```python
from build123d import *

# Parameters (mm, degrees)
SKETCH1_W           = 200
SKETCH1_H           = 42
BOSS_EXTRUDE1_DEPTH = 6.35
SKETCH4_R           = 2.286
CUT_EXTRUDE3_DEPTH  = 7.35
CHAMFER1_SIZE       = 5
SKETCH9_R           = 11
CUT_EXTRUDE8_DEPTH  = 7.35
SKETCH12_R          = 2.286
CUT_EXTRUDE11_DEPTH = 7.35
SKETCH13_R          = 2.286
SKETCH13_R_2        = 2.54
CUT_EXTRUDE12_DEPTH = 10


with BuildPart() as part:
    # Sketch1 → Boss-Extrude1 (new body)
    with BuildSketch(Plane.XY):
        Rectangle(SKETCH1_W, SKETCH1_H)
    extrude(amount=BOSS_EXTRUDE1_DEPTH)

    # Sketch4 → Cut-Extrude3 (cut, through all)
    with BuildSketch(Plane.XY.offset(6.35)):
        with Locations((-76, 0)):
            Circle(SKETCH4_R)
    extrude(amount=-CUT_EXTRUDE3_DEPTH, mode=Mode.SUBTRACT)

    # Chamfer1
    chamfer1_edges = [part.edges().sort_by_distance(p)[0] for p in [
        (100, -21, 3.175),
        (-100, -21, 3.175),
        (-100, 21, 3.175),
        (100, 21, 3.175),
    ]]
    chamfer(chamfer1_edges, length=CHAMFER1_SIZE)

    # Sketch9 → Cut-Extrude8 (cut, through all)
    with BuildSketch(Plane.XY.offset(6.35)):
        with Locations((80, 0)):
            Circle(SKETCH9_R)
    extrude(amount=-CUT_EXTRUDE8_DEPTH, mode=Mode.SUBTRACT)

    # Sketch12 → Cut-Extrude11 (cut, through all)
    with BuildSketch(Plane.XY.offset(6.35)):
        with Locations((-93, 0)):
            Circle(SKETCH12_R)
    extrude(amount=-CUT_EXTRUDE11_DEPTH, mode=Mode.SUBTRACT)

    # Sketch13 → Cut-Extrude12 (cut)
    with BuildSketch(Plane.XY.offset(6.35)):
        Polygon((-50, -16), (-50, 16), (-45, 21), (-95, 21), (-100, 16), (-100, -16), (-95, -21), (-45, -21), align=None)
        with Locations((-93, 0)):
            Circle(SKETCH13_R, mode=Mode.SUBTRACT)
        with Locations((-76, 0)):
            Circle(SKETCH13_R, mode=Mode.SUBTRACT)
        with Locations((-35, 10)):
            Circle(SKETCH13_R_2)
        with Locations((-35, -10)):
            Circle(SKETCH13_R_2)
        with Locations((-20, 10)):
            Circle(SKETCH13_R_2)
        with Locations((-20, -10)):
            Circle(SKETCH13_R_2)
        with Locations((-5, 10)):
            Circle(SKETCH13_R_2)
        with Locations((-5, -10)):
            Circle(SKETCH13_R_2)
        with Locations((10, 10)):
            Circle(SKETCH13_R_2)
        with Locations((10, -10)):
            Circle(SKETCH13_R_2)
    extrude(amount=-CUT_EXTRUDE12_DEPTH, mode=Mode.SUBTRACT)


solid = part.part
```
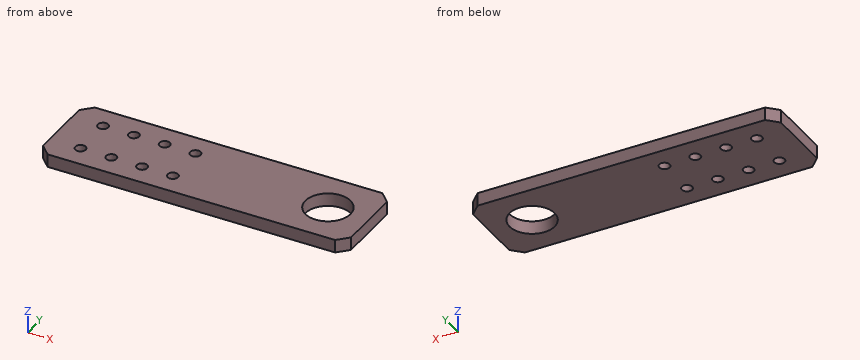
Work out the finished part from the listing and answer in its coordinate system (mm). Give positions to 0.01 mm unless a question says otherwise; leave off trailing zeros. Loops run counter-clockwise (first coordinate to the right, second up) from the corner with the lowest first, then second, coordinate; pieces in that order, holes last. Notation, with made-up numbers: (31.25, 9.5) -> (70.25, 9.5) arc R33 cw to (70.25, 47.5) -> close; hole circle Ø8 at (59.25, 49.5). An arc over 180 degrees is marked (long way). Write item = value, one per line. Start each with the question number.
(1) Find the intervals of material crossed by probe 1 along Y at (x, z) = (10, 5.25); probe 2 along X at (y, z) = (-9, 4.5); probe 3 along X at (y, z) = (-0.5, 2.5), in increasing order. Write a range as from..to.
(2) Find section C-C on z = 2.75. Give the number of separate pieces and of enclosed holes in the cut face, and give its area (3 significant figures).
(3) Find section B-B on y = 0. Give the vertices of the cut face in (x, z).
(4) Find section A-A on x = 10. Give the vertices of the cut face in (y, z).
(5) Find section D-D on x = 80. Give the vertices of the cut face in (y, z), and give its area (3 significant figures).
From the geometry:
q1.probe_1 = -21..-12.54, -7.46..7.46, 12.54..21
q1.probe_2 = -50..-37.33, -32.67..-22.33, -17.67..-7.33, -2.67..7.67, 12.33..73.68, 86.32..100
q1.probe_3 = -50..69.01, 90.99..100
q2.separate_pieces = 1
q2.enclosed_holes = 9
q2.area = 5,710 mm^2
q3.outline = (-50, 0) -> (69, 0) -> (69, 6.35) -> (-50, 6.35) -> close; (91, 0) -> (100, 0) -> (100, 6.35) -> (91, 6.35) -> close
q4.outline = (-21, 0) -> (-12.54, 0) -> (-12.54, 6.35) -> (-21, 6.35) -> close; (-7.46, 0) -> (7.46, 0) -> (7.46, 6.35) -> (-7.46, 6.35) -> close; (12.54, 0) -> (21, 0) -> (21, 6.35) -> (12.54, 6.35) -> close
q5.outline = (-21, 0) -> (-11, 0) -> (-11, 6.35) -> (-21, 6.35) -> close; (11, 0) -> (21, 0) -> (21, 6.35) -> (11, 6.35) -> close
q5.area = 127 mm^2
